The listing builds one solid part. Answer for the finished solid, in the listing's coordinates (mm). Face numbers are marked on the shaded views. Round coordinates to 2 decimals unless told otherwise and drop trailing zeros. Write each loop counter-clockwise with the first axis right and the second up, starting at its lowest first coordinate (ties: lowest second). Pieces come first, ordered by that corner, then holes.
Item 1: Find section B-B on z = 7.5. Give the vertices of the cut face in (x, y), then the cut area to 3 significant figures.
Item 2: Find the intervals of material crossed by probe 1 along X at (y, z) = (0.4, 4.5); probe 2 along X at (y, z) = (10.5, 1.5); probe 3 along Y at (x, z) = (69, 8.25), in increasing order.
Item 3: For a pull along Y with two mould halves and no side action, classify the marked faces 1 and 2 as +Y half, -Y half, draft (parallel to the pull), parting line (faces both ways), or undercut.
Item 4: Find section A-A on y = 35.5. Give the vertices of the cut face in (x, z), then the cut area to 3 significant figures.
Item 5: Each of these flat-tipped pins is pushed along its axis until it touches: pin 1 (4 mm diameter, centred on x = 60, z = 2.5, fed in from -Y); pin 2 (4 mm diameter, centred on x = 49, z = 6, fed in from -Y); pin 3 (2.5 mm diameter, centred on y = 1.5, z = 2.5, fed in from -X). Where does it stop, or does it pass through?
Item 6: Find section C-C on x = 62. Give the vertices of the cut face in (y, z).
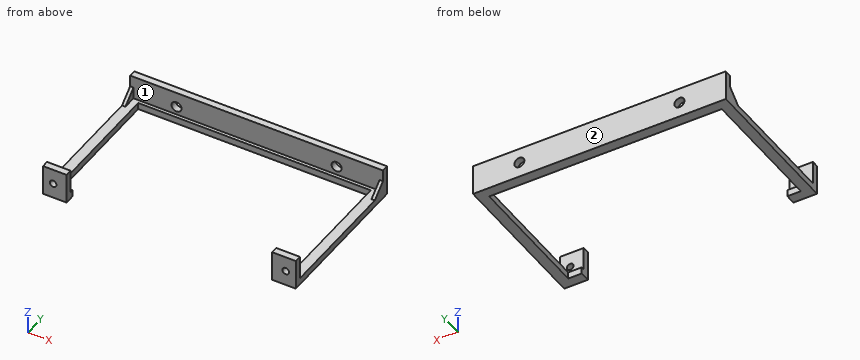
```python
from build123d import *

# Parameters (mm, degrees)
BOSS_EXTRUDE1_DEPTH = 2
BOSS_EXTRUDE2_REACH = 89.487
SKETCH2_W           = 7
SKETCH2_H           = 2
BOSS_EXTRUDE3_DEPTH = 1
CUT_EXTRUDE1_REACH  = 89.926
SKETCH7_R           = 1.5
CUT_EXTRUDE2_REACH  = 89.926
SKETCH8_R           = 1
SKETCH10_W          = 61
SKETCH10_H          = 2
CUT_EXTRUDE3_DEPTH  = 88.74394566


with BuildPart() as part:
    # Sketch1 → Boss-Extrude1 (new body)
    with BuildSketch(Plane.XY):
        Polygon((3, 3), (7, 3), (7, 0), (0, 0), (0, 45), (75, 45), (75, 0), (68, 0), (68, 3), (72, 3), (72, 42), (3, 42), align=None)
    extrude(amount=BOSS_EXTRUDE1_DEPTH)

    # Boss-Extrude2: up to this face of the body (flat: up to its plane)
    boss_extrude2_end = Plane(part.part.faces().sort_by_distance((75, 22.5, 1))[0])
    # Sketch2 → Boss-Extrude2 (add, up to the picked face)
    with BuildSketch(Plane(origin=(0, 0, 0), x_dir=(0, 0, -1), z_dir=(1, 0, 0)), mode=Mode.PRIVATE) as boss_extrude2_sk1:
        with Locations((-5.5, 44)):
            Rectangle(SKETCH2_W, SKETCH2_H)
    boss_extrude2_tool1 = split(extrude(boss_extrude2_sk1.sketch, amount=BOSS_EXTRUDE2_REACH, mode=Mode.PRIVATE), bisect_by=boss_extrude2_end, keep=Keep.BOTH, mode=Mode.PRIVATE)
    # Sketch2 → Boss-Extrude2 (add, up to the picked face)
    with BuildSketch(Plane(origin=(0, 0, 0), x_dir=(0, 0, -1), z_dir=(1, 0, 0)), mode=Mode.PRIVATE) as boss_extrude2_sk2:
        with Locations((-5.5, 1)):
            Rectangle(SKETCH2_W, SKETCH2_H)
    boss_extrude2_tool2 = split(extrude(boss_extrude2_sk2.sketch, amount=BOSS_EXTRUDE2_REACH, mode=Mode.PRIVATE), bisect_by=boss_extrude2_end, keep=Keep.BOTH, mode=Mode.PRIVATE)
    add(boss_extrude2_tool1.solids().sort_by(Axis((0, 44, 5.5), (1, 0, 0)))[0])
    add(boss_extrude2_tool2.solids().sort_by(Axis((0, 1, 5.5), (1, 0, 0)))[0])

    # Sketch5 → Boss-Extrude3 (add)
    with BuildSketch(Plane.ZY):
        Polygon((5.5, 43), (2, 39), (2, 43), align=None)
    boss_extrude3 = extrude(amount=-BOSS_EXTRUDE3_DEPTH)

    # Mirror1: Boss-Extrude3 across plane
    add(boss_extrude3.mirror(Plane.ZY.offset(-37.5)))

    # Sketch7 → Cut-Extrude1 (cut, up to next)
    with BuildSketch(Plane(origin=(0, 45, 0), x_dir=(1, 0, 0), z_dir=(0, 1, 0)), mode=Mode.PRIVATE) as cut_extrude1_sk1:
        with Locations(Location((13.750043931, -4.494608683, 0), (0, 0, 270))):
            Circle(SKETCH7_R)
    cut_extrude1_tool1 = extrude(cut_extrude1_sk1.sketch, amount=-CUT_EXTRUDE1_REACH, mode=Mode.PRIVATE) & part.part
    # Sketch7 → Cut-Extrude1 (cut, up to next)
    with BuildSketch(Plane(origin=(0, 45, 0), x_dir=(1, 0, 0), z_dir=(0, 1, 0)), mode=Mode.PRIVATE) as cut_extrude1_sk2:
        with Locations(Location((61.249956069, -4.585969821, 0), (0, 0, 270))):
            Circle(SKETCH7_R)
    cut_extrude1_tool2 = extrude(cut_extrude1_sk2.sketch, amount=-CUT_EXTRUDE1_REACH, mode=Mode.PRIVATE) & part.part
    add(cut_extrude1_tool1.solids().sort_by_distance((13.750044, 45, 4.494609))[0], mode=Mode.SUBTRACT)
    add(cut_extrude1_tool2.solids().sort_by_distance((61.249956, 45, 4.58597))[0], mode=Mode.SUBTRACT)

    # Sketch8 → Cut-Extrude2 (cut, up to next)
    with BuildSketch(Plane.XZ, mode=Mode.PRIVATE) as cut_extrude2_sk1:
        with Locations(Location((3, 4.5, 0), (0, 0, 270))):
            Circle(SKETCH8_R)
    cut_extrude2_tool1 = extrude(cut_extrude2_sk1.sketch, amount=-CUT_EXTRUDE2_REACH, mode=Mode.PRIVATE) & part.part
    # Sketch8 → Cut-Extrude2 (cut, up to next)
    with BuildSketch(Plane.XZ, mode=Mode.PRIVATE) as cut_extrude2_sk2:
        with Locations(Location((72, 4.5, 0), (0, 0, 270))):
            Circle(SKETCH8_R)
    cut_extrude2_tool2 = extrude(cut_extrude2_sk2.sketch, amount=-CUT_EXTRUDE2_REACH, mode=Mode.PRIVATE) & part.part
    add(cut_extrude2_tool1.solids().sort_by_distance((3, 0, 4.5))[0], mode=Mode.SUBTRACT)
    add(cut_extrude2_tool2.solids().sort_by_distance((72, 0, 4.5))[0], mode=Mode.SUBTRACT)

    # Sketch10 → Cut-Extrude3 (cut, through all)
    with BuildSketch(Plane(origin=(0, 0, 2), x_dir=(-1, 0, 0), z_dir=(0, 0, -1))):
        with Locations((-37.5, 1)):
            Rectangle(SKETCH10_W, SKETCH10_H)
    extrude(amount=-CUT_EXTRUDE3_DEPTH, mode=Mode.SUBTRACT)


solid = part.part
```
Check values:
1. outline: (0, 0) - (7, 0) - (7, 2) - (0, 2) - close; (0, 43) - (75, 43) - (75, 45) - (0, 45) - close; (68, 0) - (75, 0) - (75, 2) - (68, 2) - close
1. area: 178 mm2
2. probe 1: x = 0 to 2, 4 to 7, 68 to 71, 73 to 75
2. probe 2: x = 0 to 3, 72 to 75
2. probe 3: y = 0 to 2, 43 to 45
3. face 1: undercut
3. face 2: +Y half
4. outline: (0, 0) - (3, 0) - (3, 2) - (0, 2) - close; (72, 0) - (75, 0) - (75, 2) - (72, 2) - close
4. area: 12.0 mm2
5. pin 1: stops at y = 42
5. pin 2: stops at y = 43
5. pin 3: stops at x = 0
6. outline: (42, 0) - (45, 0) - (45, 3.29) - (43, 3.29) - (43, 2) - (42, 2) - close; (43, 5.88) - (45, 5.88) - (45, 9) - (43, 9) - close
